Part model, mm, in its own coordinate system. A direction names the side the tool comes from. Coordinates: 2 decimals unless noted, no trailing zeros. Loops run counter-clockwise (first coordinate to the right, second up) from the corner with the lowest first, then second, coordinate; pieces in that order, holes last. Notation, with made-up numbers: (-37.75, 64.5) -> (-16.75, 64.5) arc R21 cw to (-16.75, 74.5) -> close; hole circle Ø1 at (30, -21.5). An arc over 180 degrees is marked (long way). One line per item, written item: value. Start each with the question number.
from build123d import *

# Parameters (mm, degrees)
SKETCH2_R           = 3.175
BOSS_EXTRUDE1_DEPTH = 88.9
CHAMFER1_SIZE       = 0.9525
CUT_EXTRUDE1_DEPTH  = 3.048
SKETCH8_R           = 2.749630657
CUT_EXTRUDE2_DEPTH  = 1.27
CUT_EXTRUDE2_TAPER  = 45


with BuildPart() as part:
    # Sketch2 → Boss-Extrude1 (new body)
    with BuildSketch(Plane(origin=(44.45, 0, 0), x_dir=(0, 0, -1), z_dir=(1, 0, 0))):
        Circle(SKETCH2_R)
    extrude(amount=-BOSS_EXTRUDE1_DEPTH)

    # Chamfer1
    chamfer1_edges = [part.edges().sort_by_distance(p)[0] for p in [
        (44.45, 0, 3.175),
    ]]
    chamfer(chamfer1_edges, length=CHAMFER1_SIZE)

    # Sketch6 → Revolve1 (revolve)
    with BuildSketch(Plane.XY):
        Polygon((-50.165, 4.7625), (-50.8, 4.1275), (-50.8, 0), (-44.45, 0), (-44.45, 4.445), (-44.7675, 4.7625), align=None)
    revolve(axis=Axis((-44.45, 0, 0), (-1, 0, 0)))

    # Sketch4 → Cut-Extrude1 (cut)
    with BuildSketch(Plane(origin=(-50.8, 0, 0), x_dir=(0, 0, -1), z_dir=(1, 0, 0))):
        Polygon((0, 2.749630657), (-2.38125, 1.374815329), (-2.38125, -1.374815329), (0, -2.749630657), (2.38125, -1.374815329), (2.38125, 1.374815329), align=None)
    extrude(amount=CUT_EXTRUDE1_DEPTH, mode=Mode.SUBTRACT)

    # Sketch8 → Cut-Extrude2 (cut)
    with BuildSketch(Plane.ZY.offset(50.8)):
        Circle(SKETCH8_R)
    extrude(amount=-CUT_EXTRUDE2_DEPTH, taper=CUT_EXTRUDE2_TAPER, mode=Mode.SUBTRACT)


solid = part.part
1) Tool access for faces 4 (the flat face through (-47.752, 0, 0)), 5 (the flat face through (44.45, 0, 0)), 6 (the flat face through (-44.45, -2, 3)): list every direction of +Z, -Z, +X, -X, +Y, -Y with a clear straight run to the whole face (end or side of a thin tool).
2) Pull direction Z, two halves, no side cores. Call faces 1 (the flat face through (-50.8, 3, 1)), 2 (the cylindrical face through (0.14, -3.1, 0.69)), 3 (the flat face through (-49.297, 2.072, 1.174)): +Z half, -Z half, draft (parallel to the pull), parting line (faces both ways), or undercut.
3) Pin check, flat tips, straight feed: pin 1 Ø4 at (x, z) = (-38, 3) entering from -Y; pin 2 Ø3 at (x, z) = (-9, -1) entering from -Y (3 decimals); pin 3 Ø5 at (x, y) = (-39, 0.5) entering from +Z (3 decimals). Stop position of each tip, or through.
4) Slice it at B-B (x = -1). Give the cut face in (y, z) (3 decimals).
5) Probe line 1 (X direction, y = 2.25, z = 3.25); line 2 (X direction, y = -0.5, z = -0.5); line 3 (Z direction, x = 16, y = -0.25). List the from-to ranges inside material, lowest first. Write a range as from..to.
Check sheet entries:
1. face 4: -X
1. face 5: +Z, -Z, +X, +Y, -Y
1. face 6: +X
2. face 1: draft
2. face 2: parting line
2. face 3: undercut
3. pin 1: stops at y = -3.01
3. pin 2: stops at y = -3.175
3. pin 3: stops at z = 3.175
4. outline: circle Ø6.35 at (0, 0)
5. line 1: x = -50.8..-44.45
5. line 2: x = -47.75..44.45
5. line 3: z = -3.17..3.17
